```python
from build123d import *

# Parameters (mm, degrees)
F0_W        = 100
F0_H        = 20
F1_DEPTH    = 750
F2_R        = 47
F3_DEPTH    = 2
F4_W        = 70
F4_H        = 1470
F5_DEPTH    = 15
F6_T1_DEPTH = 70
F6_T3_DEPTH = 1470
F7_T1_DEPTH = 125
F7_T3_DEPTH = 1525
F8_T1_DEPTH = 169.300979278


# Not quite as in the source:
# - a fillet or chamfer that OpenCascade refuses, or shapes differently, is made with other operations: its cross-section is extruded or revolved along the edge and cut away or added


with BuildPart() as f1:
    # F0 (on Top) → F1 (new body, symmetric)
    with BuildSketch(Plane.XY):
        Rectangle(F0_W, F0_H)
    extrude(amount=F1_DEPTH, both=True)

    # F2 (on face) → F3 (cut)
    with BuildSketch(Plane.XZ.offset(10)):
        with Locations((0, 653)):
            Circle(F2_R)
    extrude(amount=-F3_DEPTH, mode=Mode.SUBTRACT)

    # F4 (on face) → F5 (cut)
    with BuildSketch(Plane(origin=(0, 10, 0), x_dir=(-1, 0, 0), z_dir=(0, 1, 0))):
        Rectangle(F4_W, F4_H)
    extrude(amount=-F5_DEPTH, mode=Mode.SUBTRACT)

    # F6: fillet of radius 30 on 4 edges, made by hand

    # F6_s2 → F6_t1 (join)
    with BuildSketch(Plane.YZ.offset(-35)):
        with BuildLine():
            ThreePointArc((10, 735), (-0.9807621135, 724.0192378865), (-5, 709.0192378865))
            Line((-5, 709.0192378865), (-5, 735))
            Line((-5, 735), (10, 735))
        make_face()
        with BuildLine():
            ThreePointArc((10, -735), (-0.9807621135, -724.0192378865), (-5, -709.0192378865))
            Line((-5, -709.0192378865), (-5, -735))
            Line((-5, -735), (10, -735))
        make_face()
    extrude(amount=F6_T1_DEPTH)

    # F6_s4 → F6_t3 (join)
    with BuildSketch(Plane.XY.offset(-735)):
        with BuildLine():
            ThreePointArc((35, 10), (24.0192378865, -0.9807621135), (9.0192378865, -5))
            Line((9.0192378865, -5), (35, -5))
            Line((35, -5), (35, 10))
        make_face()
        with BuildLine():
            ThreePointArc((-35, 10), (-24.0192378865, -0.9807621135), (-9.0192378865, -5))
            Line((-9.0192378865, -5), (-35, -5))
            Line((-35, -5), (-35, 10))
        make_face()
    extrude(amount=F6_T3_DEPTH)

    # F7: fillet of radius 5 on 5 edges, made by hand

    # F7_s2 → F7_t1 (cut)
    with BuildSketch(Plane.YZ.offset(-62.5)):
        with BuildLine():
            ThreePointArc((-10, -745), (-8.5355339059, -748.5355339059), (-5, -750))
            Line((-5, -750), (-10, -750))
            Line((-10, -750), (-10, -745))
        make_face()
        with BuildLine():
            ThreePointArc((-10, 745), (-8.5355339059, 748.5355339059), (-5, 750))
            Line((-5, 750), (-10, 750))
            Line((-10, 750), (-10, 745))
        make_face()
    extrude(amount=F7_T1_DEPTH, mode=Mode.SUBTRACT)

    # F7_s4 → F7_t3 (cut)
    with BuildSketch(Plane.XY.offset(-762.5)):
        with BuildLine():
            ThreePointArc((-45, -10), (-48.5355339059, -8.5355339059), (-50, -5))
            Line((-50, -5), (-50, -10))
            Line((-50, -10), (-45, -10))
        make_face()
        with BuildLine():
            ThreePointArc((45, -10), (48.5355339059, -8.5355339059), (50, -5))
            Line((50, -5), (50, -10))
            Line((50, -10), (45, -10))
        make_face()
    extrude(amount=F7_T3_DEPTH, mode=Mode.SUBTRACT)

    # F7_s5 → F7_t6 (revolve, cut)
    with BuildSketch(Plane.XY.offset(653)):
        with BuildLine():
            ThreePointArc((51, -10), (48.7639320225, -9.472135955), (47, -8))
            Line((47, -8), (47, -10))
            Line((47, -10), (51, -10))
        make_face()
    revolve(axis=Axis((0, -10, 653), (0, -1, 0)), mode=Mode.SUBTRACT)

    # F8: chamfer of 30 on 2 edges, made by hand

    # F8_s2 → F8_t1 (cut)
    with BuildSketch(Plane.XZ.offset(-87.150489639)):
        Polygon((50, -720), (20, -750), (50, -750), align=None)
        Polygon((-50, -720), (-20, -750), (-50, -750), align=None)
    extrude(amount=F8_T1_DEPTH, mode=Mode.SUBTRACT)


solid = f1.part
```
For this review, take the finished solid that the model builds, in its own axes (mm). A direction names the side the tool comes from. Coordinates: 2 decimals unless noted, no trailing zeros. Loops run counter-clockwise (first coordinate to the right, second up) from the corner with the lowest first, then second, coordinate; pieces in that order, holes last.
1. Add section B-B, the plane y = 4.5. Give the boundary of the cut face in (x, z), then the cut area to 3 significant figures.
2. Mouldability with a two-part tool opening along X and no side actions: class faces 1 (the flat face through (-35, 0, -735)), 2 (the flat face through (-1, -10, -48)), 3 (the cylindrical face through (24.21, -0.87, -10.29)) as +X half, -X half, draft (parallel to the pull), parting line (faces both ways), or undercut.
3. For line 1 (X direction, y = -0.5, z = -456); line 2 (Y direction, x = -0.5, z = -406.5); line 3 (Y direction, x = 11.5, z = 262), list the stretches that pass through material, from the lowest coordinate up.
4. Add section A-A, the plane z = 543.5. Give the boundary of the cut face in (x, y), then the cut area to 3 significant figures.
5. For faces 4 (the flat face through (35, 0, -735)), 5 (the cylindrical face through (-0.49, 1.07, 727.11)), 6 (the flat face through (-1, -8, 654)), list the 3-axis set-ups (+Z, -Z, +X, -X, +Y, -Y) from which the entire face can be reached by the end or side of a thin tool; tool diameter is ignored.
6. Insertion check: P1, Ø6, axis at x = -13, z = -293.5, coming from the +Y side; P2, Ø3, axis at x = 5.5, z = 86, coming from the +Y side. Each pin has a flat end and moves straight along its axis. Give the tip position at first contact, or say it passes through.
Result:
1. outline: (-50, -720) - (-20, -750) - (20, -750) - (50, -720) - (50, 750) - (-50, 750) - close; hole (-30.92, -730.92) - (30.92, -730.92) - (30.92, 730.92) - (-30.92, 730.92) - close
1. area: 58,700 mm2
2. face 1: -X half
2. face 2: draft
2. face 3: undercut
3. line 1: x = -50 to -24.82, 24.82 to 50
3. line 2: y = -10 to -5
3. line 3: y = -10 to -4.9
4. outline: (-50, -5) arc R5 ccw to (-45, -10) - (45, -10) arc R5 ccw to (50, -5) - (50, 10) - (35, 10) arc R30 cw to (9.02, -5) - (-9.02, -5) arc R30 cw to (-35, 10) - (-50, 10) - close
4. area: 1,170 mm2
5. face 4: -Z, +X, +Y, -Y
5. face 5: +Y
5. face 6: -Y
6. P1: stops at y = -4.18
6. P2: stops at y = -5
